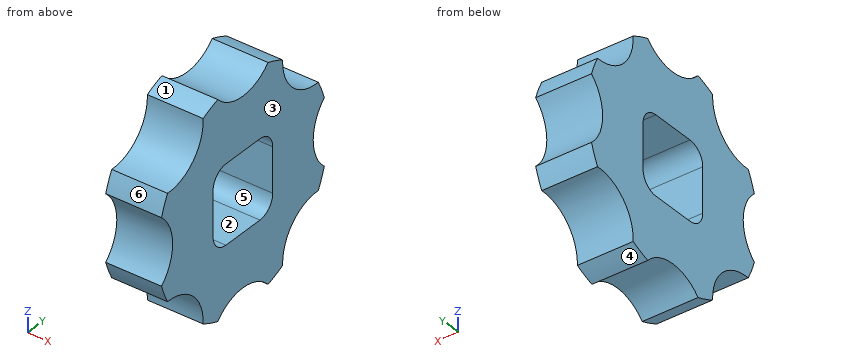
from build123d import *

# Parameters (mm, degrees)
SKETCH1_R           = 20
BOSS_EXTRUDE1_DEPTH = 10
SKETCH2_W           = 14
SKETCH2_H           = 14
CUT_EXTRUDE1_DEPTH  = 10
FILLET1_R           = 3
SKETCH3_R           = 8
CUT_EXTRUDE2_DEPTH  = 10
SKETCH3_3_R         = 8
CUT_EXTRUDE3_DEPTH  = 10
CIRPATTERN2_COUNT   = 8


with BuildPart() as part:
    # Sketch1 → Boss-Extrude1 (new body)
    with BuildSketch(Plane(origin=(0, 0, 0), x_dir=(0, 0, -1), z_dir=(1, 0, 0))):
        Circle(SKETCH1_R)
    extrude(amount=BOSS_EXTRUDE1_DEPTH)

    # Sketch2 → Cut-Extrude1 (cut)
    with BuildSketch(Plane(origin=(10, 0, 0), x_dir=(0, 0, -1), z_dir=(1, 0, 0))):
        Rectangle(SKETCH2_W, SKETCH2_H)
    extrude(amount=-CUT_EXTRUDE1_DEPTH, mode=Mode.SUBTRACT)

    # Fillet1
    fillet1_edges = [part.edges().sort_by_distance(p)[0] for p in [
        (5, 7, 7),
        (5, 7, -7),
        (5, -7, -7),
        (5, -7, 7),
    ]]
    fillet(fillet1_edges, radius=FILLET1_R)

    # Sketch3 → Cut-Extrude2 (cut)
    with BuildSketch(Plane(origin=(10, 0, 0), x_dir=(0, 0, -1), z_dir=(1, 0, 0))):
        with Locations((-24.5, 0)):
            Circle(SKETCH3_R)
    cut_extrude2 = extrude(amount=-CUT_EXTRUDE2_DEPTH, mode=Mode.SUBTRACT)

    # Sketch3_3 → Cut-Extrude3 (cut)
    with BuildSketch(Plane(origin=(10, 0, 0), x_dir=(0, 0, -1), z_dir=(1, 0, 0))):
        with Locations((24.5, 0)):
            Circle(SKETCH3_3_R)
        with Locations((-24.5, 0)):
            Circle(SKETCH3_3_R)
    extrude(amount=-CUT_EXTRUDE3_DEPTH, mode=Mode.SUBTRACT)

    # CirPattern2: Cut-Extrude2 ×8 about axis
    cirpattern2_axis = Axis((0, 0, 0), (1, 0, 0))
    for i in range(1, CIRPATTERN2_COUNT):
        add(cut_extrude2.rotate(cirpattern2_axis, i * 360 / CIRPATTERN2_COUNT), mode=Mode.SUBTRACT)


solid = part.part
Can you work these out from the model? Positions are in its coordinate system, mm. Face numbers are marked on the shaded views. A direction names the side the tool comes from. Coordinates: 2 decimals unless noted, no trailing zeros. Loops run counter-clockwise (first coordinate to the right, second up) from the corner with the lowest first, then second, coordinate; pieces in that order, holes last. Notation, with made-up numbers: M 74,-10 L 101,-10 A8 ccw 101,-4 Z; hole C 52,13.25 d3. An arc over 180 degrees is marked long. Answer as CSV lines item,"result". Start each with the question number.
1. Suppose I cut it at B-B, the plane z = -3.5. List the corners of the cut face in (x, y) for me.
2. If I drill on probe 1 along Z at (x, y) = (5, 0); probe 2 along Z at (x, y) = (4.75, 5) (3 decimals); probe 3 along Y at (x, z) = (4.5, -4.5), over which ranges is the centre line in solid material (lowest first)? Write a range as [from, to].
3. Thinking about a two-plate mould opening in Z: for the marked faces 3, 4, 5 and 6, which applies, +Z half, -Z half, draft (parallel to the pull), parting line (faces both ways), or undercut?
4. For pin 1 Ø2.5 at (x, z) = (2.5, 0.5) entering from -Y; pin 2 Ø1.5 at (x, y) = (8.5, 6) entering from -Z; pin 3 Ø2 at (x, y) = (7.5, 1) entering from -Z; pin 4 Ø2.5 at (x, y) = (3, -1.5) entering from +Z, each with a flat end and sliding along its axis, tell me the tip position at first contact or that it passes through.
5. Suppose I cut it at A-A, the plane x = 1. List the corners of the cut face in (y, z) for me, plus the area to 3 significant figures.
6. Suppose I cut it at C-C, the plane y = 5. List the corners of the cut face in (x, z) for me (3 decimals).
7. Suppose I cut it at D-D, the plane z = -13.5. List the corners of the cut face in (x, y) for me.
8. For the marked faces 1 and 2, which set-ups out of +Z, -Z, +X, -X, +Y, -Y let a thin tool reach every point of the face, with its end or its side?
Output:
1,outline,"M 0,-17.31 L 10,-17.31 L 10,-7 L 0,-7 Z; M 0,7 L 10,7 L 10,17.31 L 0,17.31 Z"
2,probe 1,"z = [-16.5, -7], [7, 16.5]"
2,probe 2,"z = [-18.255, -6.828], [6.828, 18.255]"
2,probe 3,"y = [-17.89, -6.96], [6.96, 17.89]"
3,face 3,"draft"
3,face 4,"-Z half"
3,face 5,"undercut"
3,face 6,"+Z half"
4,pin 1,"stops at y = -16.69"
4,pin 2,"stops at z = -19.11"
4,pin 3,"stops at z = -16.75"
4,pin 4,"stops at z = 16.99"
5,outline,"M -19.11,-5.91 A20 ccw -17.69,-9.33 A8 cw -9.33,-17.69 A20 ccw -5.91,-19.11 A8 cw 5.91,-19.11 A20 ccw 9.33,-17.69 A8 cw 17.69,-9.33 A20 ccw 19.11,-5.91 A8 cw 19.11,5.91 A20 ccw 17.69,9.33 A8 cw 9.33,17.69 A20 ccw 5.91,19.11 A8 cw -5.91,19.11 A20 ccw -9.33,17.69 A8 cw -17.69,9.33 A20 ccw -19.11,5.91 A8 cw Z; hole M -7,-4 A3 ccw -4,-7 L 4,-7 A3 ccw 7,-4 L 7,4 A3 ccw 4,7 L -4,7 A3 ccw -7,4 Z"
5,area,"841 mm^2"
6,outline,"M 0,-18.255 L 10,-18.255 L 10,-6.828 L 0,-6.828 Z; M 0,6.828 L 10,6.828 L 10,18.255 L 0,18.255 Z"
7,outline,"M 0,-10.3 L 10,-10.3 L 10,10.3 L 0,10.3 Z"
8,face 1,"+Z, +X, -X, -Y"
8,face 2,"+X, -X"
